Here's how the part is built. I have some questions about the finished solid (model axes, mm). A direction names the side the tool comes from. Coordinates: 2 decimals unless noted, no trailing zeros. Write each loop counter-clockwise with the first axis right and the second up, starting at its lowest first coordinate (ties: lowest second). Pieces come first, ordered by that corner, then holes.
```python
from build123d import *

# Parameters (mm, degrees)
SKETCH1_R           = 49
BOSS_EXTRUDE1_DEPTH = 15
SKETCH7_R           = 5
CUT_EXTRUDE1_DEPTH  = 71.901339903
SKETCH8_R           = 25
BOSS_EXTRUDE2_DEPTH = 60
SKETCH10_R          = 15
SKETCH10_R_2        = 30
SKETCH10_R_3        = 25
BOSS_EXTRUDE3_DEPTH = 15
SKETCH11_R          = 6
CUT_EXTRUDE3_DEPTH  = 33
SKETCH11_3_R        = 6
SKETCH11_3_R_2      = 17.5
CUT_EXTRUDE4_DEPTH  = 30
SKETCH12_R          = 13
CUT_EXTRUDE5_DEPTH  = 60


with BuildPart() as part:
    # Sketch1 → Boss-Extrude1 (new body)
    with BuildSketch(Plane.XY):
        Circle(SKETCH1_R)
    extrude(amount=BOSS_EXTRUDE1_DEPTH)

    # Sketch7 → Cut-Extrude1 (cut, through all)
    with BuildSketch(Plane.XY.offset(15)):
        with Locations((0, 35)):
            Circle(SKETCH7_R)
        with Locations((30.310889132, 17.5)):
            Circle(SKETCH7_R)
        with Locations((30.310889132, -17.5)):
            Circle(SKETCH7_R)
        with Locations((0, -35)):
            Circle(SKETCH7_R)
        with Locations((-30.310889132, -17.5)):
            Circle(SKETCH7_R)
        with Locations((-30.310889132, 17.5)):
            Circle(SKETCH7_R)
    extrude(amount=-CUT_EXTRUDE1_DEPTH, mode=Mode.SUBTRACT)

    # Sketch8 → Boss-Extrude2 (add)
    with BuildSketch(Plane.XY.offset(15)):
        Circle(SKETCH8_R)
    extrude(amount=BOSS_EXTRUDE2_DEPTH)

    # Sketch10 → Boss-Extrude3 (add)
    # profile 1 of 6: a face of its own
    with BuildSketch(Plane.XY.offset(75)):
        with Locations((0, 50)):
            Circle(SKETCH10_R)
    # profile 2 of 6: a face of its own
    with BuildSketch(Plane.XY.offset(75)):
        with BuildLine():
            Line((-14.309088021, 54.5), (-28.618176043, 9))
            ThreePointArc((-28.618176043, 9), (0, 30), (28.618176043, 9))
            Line((28.618176043, 9), (14.309088021, 54.5))
            ThreePointArc((14.309088021, 54.5), (14.826265887, 52.276365489), (15, 50))
            ThreePointArc((15, 50), (-2.276365489, 35.173734113), (-14.309088021, 54.5))
        make_face()
    # profile 3 of 6: a face of its own
    with BuildSketch(Plane.XY.offset(75)):
        with Locations((0, -50)):
            Circle(SKETCH10_R)
    # profile 4 of 6: a face of its own
    with BuildSketch(Plane.XY.offset(75)):
        with BuildLine():
            Line((14.309088021, -54.5), (28.618175991, -9.000000163))
            ThreePointArc((28.618175991, -9.000000163), (-8.5e-08, -30), (-28.618176043, -9))
            Line((-28.618176043, -9), (-14.309088021, -54.5))
            ThreePointArc((-14.309088021, -54.5), (-2.276365489, -35.173734113), (15, -50))
            ThreePointArc((15, -50), (14.826265887, -52.276365489), (14.309088021, -54.5))
        make_face()
    # profile 5 of 6: a face of its own
    with BuildSketch(Plane.XY.offset(75)):
        Circle(SKETCH10_R_2)
        Circle(SKETCH10_R_3, mode=Mode.SUBTRACT)
    # profile 6 of 6: a face of its own
    with BuildSketch(Plane.XY.offset(75)):
        Circle(SKETCH10_R_3)
    extrude(amount=BOSS_EXTRUDE3_DEPTH)

    # Sketch11 → Cut-Extrude3 (cut)
    with BuildSketch(Plane.XY.offset(90)):
        with Locations((0, 50)):
            Circle(SKETCH11_R)
        with Locations((0, -50)):
            Circle(SKETCH11_R)
    extrude(amount=-CUT_EXTRUDE3_DEPTH, mode=Mode.SUBTRACT)

    # Sketch11_3 → Cut-Extrude4 (cut)
    with BuildSketch(Plane.XY.offset(90)):
        with Locations((0, 50)):
            Circle(SKETCH11_3_R)
        with Locations((0, -50)):
            Circle(SKETCH11_3_R)
        Circle(SKETCH11_3_R_2)
    extrude(amount=-CUT_EXTRUDE4_DEPTH, mode=Mode.SUBTRACT)

    # Sketch12 → Cut-Extrude5 (cut)
    with BuildSketch(Plane(origin=(0, 0, 0), x_dir=(-1, 0, 0), z_dir=(0, 0, -1))):
        Circle(SKETCH12_R)
    extrude(amount=-CUT_EXTRUDE5_DEPTH, mode=Mode.SUBTRACT)


solid = part.part
```
1) Imagine slicing it at A-A on y = 0. Please give me the cut outline in (x, z).
Values follow:
outline: (-49, 0) - (-13, 0) - (-13, 60) - (-17.5, 60) - (-17.5, 90) - (-30, 90) - (-30, 75) - (-25, 75) - (-25, 15) - (-49, 15) - close; (13, 0) - (49, 0) - (49, 15) - (25, 15) - (25, 75) - (30, 75) - (30, 90) - (17.5, 90) - (17.5, 60) - (13, 60) - close
2) We'd pull the mould along X, two halves only. Please class faces 1 (the face through (3, 39, 8)), 2 (the face through (29.23, 12.62, 7.6)), 3 (the face through (0, -65, 82)), 4 (the face through (-11.6, 22.5, 15)): pulls with the +X half, pulls with the -X half, needs draft (parallel to the pull), parting line crosses it, or undercut.
Values follow:
face 1: undercut
face 2: undercut
face 3: parting line crosses it
face 4: needs draft
3) Imagine slicing it at D-D on x = -8. Please give me the cut outline in (y, z).
Values follow:
outline: (-62.69, 75) - (-23.69, 75) - (-23.69, 15) - (-48.34, 15) - (-48.34, 0) - (-10.25, 0) - (-10.25, 60) - (-15.56, 60) - (-15.56, 90) - (-62.69, 90) - close; (10.25, 0) - (48.34, 0) - (48.34, 15) - (23.69, 15) - (23.69, 75) - (62.69, 75) - (62.69, 90) - (15.56, 90) - (15.56, 60) - (10.25, 60) - close
4) On a 3-axis mill with a long thin cutter (end or side, diameter ignored), from which of +Z, -Z, +X, -X, +Y, -Y can I reach the whole of each face in a straight line? I mean faces 5 (the face through (-30, 0, 82)), 6 (the face through (26.34, 41.32, 7.4)), 7 (the face through (23.846, 7.509, 44.58)), 8 (the face through (-1.301, -55.857, 82.605)). Say none if no direction works.
Values follow:
face 5: +Z, -X
face 6: -Z
face 7: none
face 8: +Z
5) Imagine slicing it at C-C on y = -20. Please give me the cut outline in (x, z).
Values follow:
outline: (-44.73, 0) - (-34.64, 0) - (-34.64, 15) - (-44.73, 15) - close; (-25.98, 0) - (25.98, 0) - (25.98, 15) - (15, 15) - (15, 75) - (25.16, 75) - (25.16, 90) - (-25.16, 90) - (-25.16, 75) - (-15, 75) - (-15, 15) - (-25.98, 15) - close; (34.64, 0) - (44.73, 0) - (44.73, 15) - (34.64, 15) - close
6) Imagine slicing it at B-B on z = 76.5. Please give me the cut outline in (x, y), then the cut area to 3 significant figures.
Values follow:
outline: (-28.62, -9) - (-14.31, -54.5) arc R15 ccw to (14.31, -54.5) - (28.62, -9) arc R30 ccw to (28.62, 9) - (14.31, 54.5) arc R15 ccw to (-14.31, 54.5) - (-28.62, 9) arc R30 ccw to start; hole circle Ø35 at (0, 0); hole circle Ø12 at (0, -50); hole circle Ø12 at (0, 50)
area: 4,220 mm2
7) Will these pins go through, and if not, where does the flat tip stop? pin 1 (7 mm diameter, centred on x = 0, y = 50, fed in from -Z); pin 2 (12 mm diameter, centred on x = 35.5, y = -11, fed in from +Z); pin 3 (3 mm diameter, centred on y = -19.5, z = 25.5, fed in from -X); pin 4 (2 mm diameter, centred on x = 16, z = 70.5, fed in from +Y).
Values follow:
pin 1: stops at z = 0
pin 2: stops at z = 15
pin 3: stops at x = -17.35
pin 4: stops at y = 20
8) I need wall thicknesses on probe 1 along X at (y, z) = (-17, 7); probe 2 along Z at (x, y) = (-44.5, -19); probe 3 along Z at (x, y) = (27, 6.5). Which ranges of each line are inside material? Lowest first, please.
Values follow:
probe 1: x = -45.96 to -35.29, -25.34 to 25.34, 35.29 to 45.96
probe 2: z = 0 to 15
probe 3: z = 0 to 15, 75 to 90
